Design review of the part shown in the three views and the two pictorial views. Dimensions are in mm from the part's minimum x, y and z. Round coordinates to 2 decimals unless told otherwise and drop trailing zeros. Write each loop counter-clockwise with the first axis right and the second up, starting at its lowest first coordinate (ties: lowest second). Pieces come first, ordered by that corner, then holes. Notation, with made-up numbers: (42.5, -29) - (77.5, -29) arc R6 ccw to (77.5, -19) - close; hole circle Ø4 at (-40, 52). An arc over 180 degrees is marked (long way). One line per item, written item: value. Start each with the question number.
Q1. Clearance check with flat-ended pins moving along their axes: pin 1 Ø6 at (x, z) = (23.5, 21.5) entering from -Y (1 decimal); pin 2 Ø5 at (x, z) = (16.5, 42.5) entering from +Y (3 decimals); pin 3 Ø10 at (y, z) = (6, 59.5) entering from -X; pin 4 Ø3 at (x, z) = (25, 18.5) entering from -Y. State where each tip first meets the part, or that it passes through.
Q2. Add section C-C on z = 46. Write out the cut boundary in (x, y).
Q3. For probe 1 along Y at (x, z) = (20, 58.5); probe 2 along Y at (x, z) = (34, 61.5) (1 decimal); probe 3 along X at (y, z) = (7.5, 54.5), list the stretches that pass through material, from the lowest coordinate up.
Q4. Mouldability with a two-part tool opening along X and no side actions: class the marked faces 1 and 2 as +X half, -X half, draft (parallel to the pull), parting line (faces both ways), or undercut.
Q5. Add section A-A on x = 20. Write out the cut boundary in (y, z).
Q6. Add section D-D on z = 26. Write out the cut boundary in (x, y).
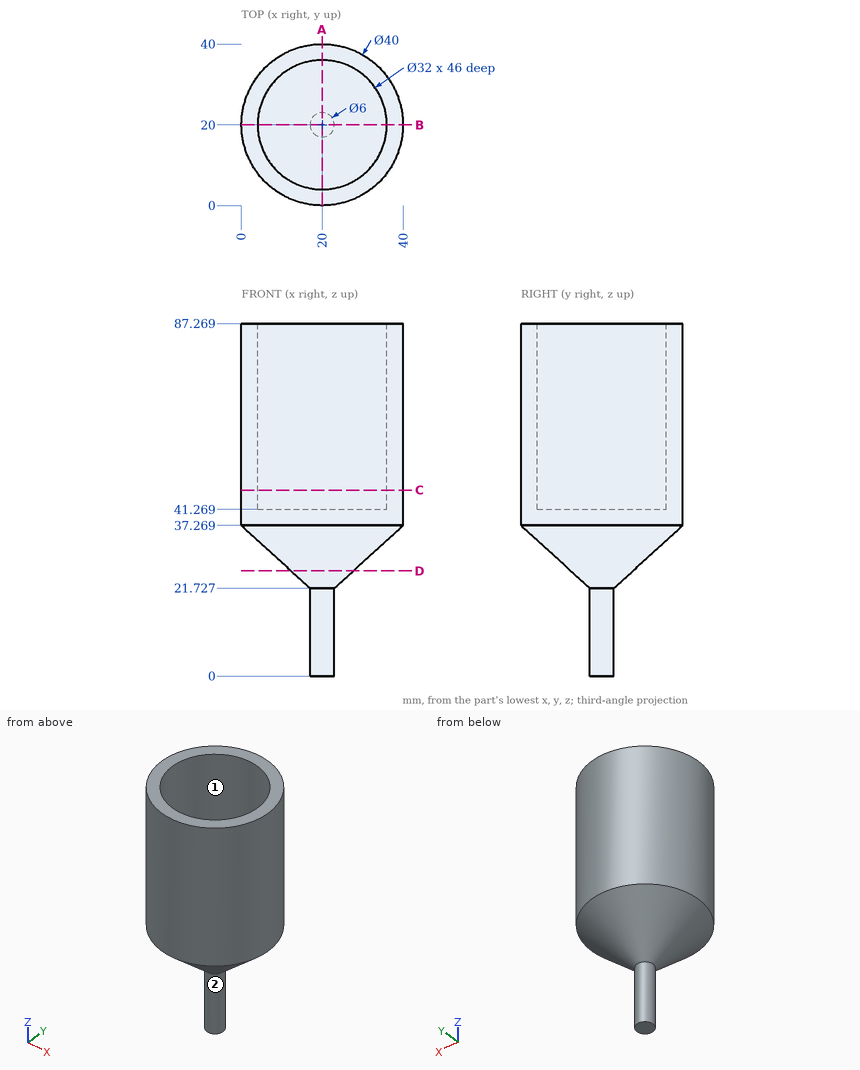
Result set:
1. pin 1: stops at y = 14.7
1. pin 2: stops at y = 39.975
1. pin 3: stops at x = 2.14
1. pin 4: passes through
2. outline: circle Ø40 at (20, 20); hole circle Ø32 at (20, 20)
3. probe 1: y = 0 to 4, 36 to 40
3. probe 2: y = 5.7 to 12.3, 27.7 to 34.3
3. probe 3: x = 4.39 to 10.01, 29.99 to 35.61
4. face 1: undercut
4. face 2: parting line
5. outline: (0, 37.27) - (17, 21.73) - (17, 0) - (23, 0) - (23, 21.73) - (40, 37.27) - (40, 87.27) - (36, 87.27) - (36, 41.27) - (4, 41.27) - (4, 87.27) - (0, 87.27) - close
6. outline: circle Ø15.35 at (20, 20)
